The model under review builds one solid part; all positions refer to its coordinate system, in mm. Face numbers are marked on the shaded views. Round coordinates to 2 decimals unless told otherwise and drop trailing zeros. Write each loop counter-clockwise with the first axis right and the second up, starting at its lowest first coordinate (ties: lowest second). Pieces come first, ordered by that corner, then holes. Notation, with made-up numbers: M -10.75,31 L 12.25,31 A18 ccw 12.25,63 Z; hole C 65,-29.75 d4. An arc over 180 degrees is marked long. Write item = value, one per line. Start each with the question number.
Item 1: Take a section at C-C, the plane x = 54. Give the boundary of the cut face in (y, z), plus the area to 3 significant figures.
Item 2: Take a section at A-A, the plane y = 101. Give the boundary of the cut face in (x, z), plus the area to 3 significant figures.
Item 3: The part is to be moulded in two halves that separate along X. For the marked faces 1, 2 and 3, say which applies: +X half, -X half, draft (parallel to the pull), parting line (faces both ways), or undercut.
Item 4: Take a section at B-B, the plane y = 39. Give the boundary of the cut face in (x, z).
Item 5: For pin 1 Ø2 at (x, y) = (28, 55) entering from +Z; pin 2 Ø10 at (x, y) = (10, 46) entering from -Z; pin 3 Ø3 at (x, z) = (2.5, 6) entering from -Y; pin 4 Ø1.5 at (x, y) = (6, 39) entering from +Z, all flat-tipped, find the tip position at first contact; note any pin that passes through.
Item 6: Take a section at D-D, the plane x = 28.5. Give the boundary of the cut face in (y, z), plus the area to 3 significant figures.
Item 7: To check wall thickness, follow line 1 along Y through (x, z) = (30, 1.3); line 2 along X through (y, z) = (115.5, 2.5); line 3 along Z through (x, y) = (22.5, 76.5). State the ranges of each line that lie inside material, in increasing order.
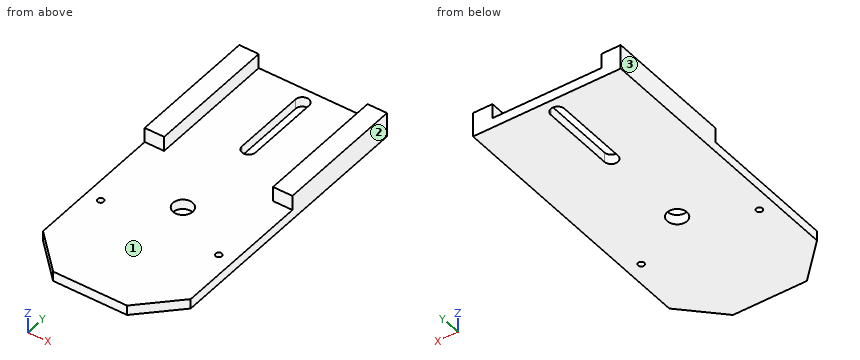
from build123d import *

# Parameters (mm, degrees)
ESQUISSE1_W             = 60
ESQUISSE1_H             = 125
BOSS_EXTRU_1_DEPTH      = 10
ESQUISSE2_R             = 4
ENL_V_MAT_EXTRU_1_DEPTH = 11
ESQUISSE4_W             = 6
ESQUISSE4_H             = 72
ENL_V_MAT_EXTRU_2_DEPTH = 61
TROU_TARAUD_M33_D       = 2.5
TROU_TARAUD_M34_D       = 2.5
CHANFREIN1_SIZE         = 15
ESQUISSE15_W            = 44.2
ESQUISSE15_H            = 6
ENL_V_MAT_EXTRU_4_DEPTH = 55
ENL_V_MAT_EXTRU_5_DEPTH = 11


with BuildPart() as part:
    # Esquisse1 → Boss.-Extru.1 (new body)
    with BuildSketch(Plane.XY):
        with Locations((30, 62.5)):
            Rectangle(ESQUISSE1_W, ESQUISSE1_H)
    extrude(amount=BOSS_EXTRU_1_DEPTH)

    # Esquisse2 → Enlèv. mat.-Extru.1 (cut, through all)
    with BuildSketch(Plane.XY.offset(10)):
        with Locations((30, 52)):
            Circle(ESQUISSE2_R)
    extrude(amount=-ENL_V_MAT_EXTRU_1_DEPTH, mode=Mode.SUBTRACT)

    # Esquisse4 → Enlèv. mat.-Extru.2 (cut, through all)
    with BuildSketch(Plane.ZY):
        with Locations((7, 36)):
            Rectangle(ESQUISSE4_W, ESQUISSE4_H)
    extrude(amount=-ENL_V_MAT_EXTRU_2_DEPTH, mode=Mode.SUBTRACT)

    # Trou taraudé M33 (through all)
    with Locations(Plane.XY.offset(4)):
        with Locations((54, 39)):
            Hole(TROU_TARAUD_M33_D / 2)

    # Trou taraudé M34 (through all)
    with Locations(Plane.XY.offset(4)):
        with Locations((6, 39)):
            Hole(TROU_TARAUD_M34_D / 2)

    # Chanfrein1
    chanfrein1_edges = [part.edges().sort_by_distance(p)[0] for p in [
        (60, 0, 2),
        (0, 0, 2),
    ]]
    chamfer(chanfrein1_edges, length=CHANFREIN1_SIZE)

    # Esquisse15 → Enlèv. mat.-Extru.4 (cut)
    with BuildSketch(Plane(origin=(0, 125, 0), x_dir=(1, 0, 0), z_dir=(0, 1, 0))):
        with Locations((30, -7)):
            Rectangle(ESQUISSE15_W, ESQUISSE15_H)
    extrude(amount=-ENL_V_MAT_EXTRU_4_DEPTH, mode=Mode.SUBTRACT)

    # Esquisse16 → Enlèv. mat.-Extru.5 (cut, through all)
    with BuildSketch(Plane(origin=(0, 0, 0), x_dir=(-1, 0, 0), z_dir=(0, 0, -1))):
        with BuildLine():
            Line((-27.202577742, 119), (-27.202577742, 89))
            ThreePointArc((-27.202577742, 89), (-29.952577742, 86.25), (-32.702577742, 89))
            Line((-32.702577742, 89), (-32.702577742, 119))
            ThreePointArc((-32.702577742, 119), (-29.952577742, 121.75), (-27.202577742, 119))
        make_face()
    extrude(amount=-ENL_V_MAT_EXTRU_5_DEPTH, mode=Mode.SUBTRACT)


solid = part.part
Response values:
q1.outline = M 9,0 L 37.75,0 L 37.75,4 L 9,4 Z; M 40.25,0 L 125,0 L 125,10 L 72,10 L 72,4 L 40.25,4 Z
q1.area = 772 mm2
q2.outline = M 0,0 L 27.2,0 L 27.2,4 L 7.9,4 L 7.9,10 L 0,10 Z; M 32.7,0 L 60,0 L 60,10 L 52.1,10 L 52.1,4 L 32.7,4 Z
q2.area = 313 mm2
q3.face_1 = undercut
q3.face_2 = +X half
q3.face_3 = -X half
q4.outline = M 0,0 L 4.75,0 L 4.75,4 L 0,4 Z; M 7.25,0 L 52.75,0 L 52.75,4 L 7.25,4 Z; M 55.25,0 L 60,0 L 60,4 L 55.25,4 Z
q5.pin_1 = 4
q5.pin_2 = 0
q5.pin_3 = 72
q5.pin_4 = through
q6.outline = M 0,0 L 48.29,0 L 48.29,4 L 0,4 Z; M 55.71,0 L 86.66,0 L 86.66,4 L 55.71,4 Z; M 121.34,0 L 125,0 L 125,4 L 121.34,4 Z
q6.area = 332 mm2
q7.line_1 = 0 to 48, 56 to 86.25, 121.75 to 125
q7.line_2 = 0 to 27.2, 32.7 to 60
q7.line_3 = 0 to 4
